CAD build for the part. Positions are in the model's coordinates, mm. Face numbers are marked on the shaded views. Round coordinates to 2 decimals unless told otherwise and drop trailing zeros. Loops run counter-clockwise (first coordinate to the right, second up) from the corner with the lowest first, then second, coordinate; pieces in that order, holes last.
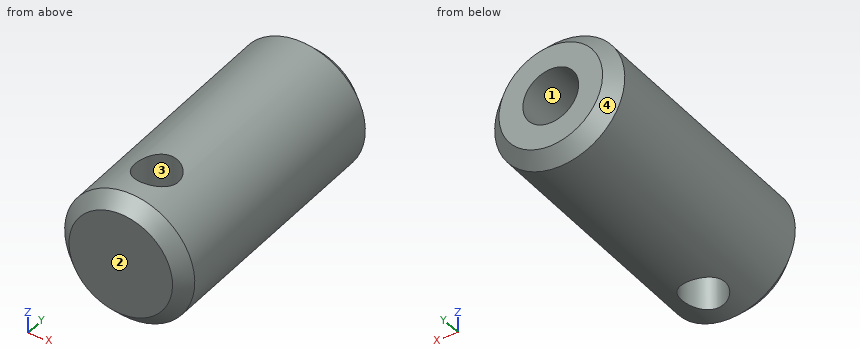
from build123d import *

# Parameters (mm, degrees)
SKETCH_1_R             = 4.9
EXTRUDE_1_DEPTH        = 21
HOLE_WIZARD_M4_1_D     = 3.3
HOLE_WIZARD_M5_1_D     = 4.2
HOLE_WIZARD_M5_1_DEPTH = 12
HOLE_WIZARD_M5_1_TIP   = 1.2618073
CHAMFER_1_SIZE         = 1


with BuildPart() as part:
    # 草图1 → 凸台-拉伸1 (new body)
    with BuildSketch(Plane(origin=(0, 0, 0), x_dir=(1, 0, 0), z_dir=(0, 1, 0))):
        with Locations(Location((0, 0, 0), (0, 0, 90))):
            Circle(SKETCH_1_R)
    extrude(amount=EXTRUDE_1_DEPTH)

    # M4 螺纹孔1 (through all)
    with Locations(Plane.XY.offset(4.9)):
        with Locations((0, 4)):
            Hole(HOLE_WIZARD_M4_1_D / 2)

    # M5 螺纹孔1
    with Locations(Plane(origin=(0, 21, 0), x_dir=(1, 0, 0), z_dir=(0, 1, 0))):
        with Locations((0, 0)):
            Hole(HOLE_WIZARD_M5_1_D / 2, depth=HOLE_WIZARD_M5_1_DEPTH)
            with Locations((0, 0, -(HOLE_WIZARD_M5_1_DEPTH + HOLE_WIZARD_M5_1_TIP / 2))):  # 118° drill point
                Cone(0, HOLE_WIZARD_M5_1_D / 2, HOLE_WIZARD_M5_1_TIP, mode=Mode.SUBTRACT)

    # 倒角1
    chamfer_1_edges = [part.edges().sort_by_distance(p)[0] for p in [
        (0, 0, 4.9),
        (0, 21, 4.9),
    ]]
    chamfer(chamfer_1_edges, length=CHAMFER_1_SIZE)


solid = part.part
Item 1: Cut at B-B (y = 4). List the corners of the cut face in (x, z), plus the area to 3 significant figures.
Verdict:
outline: (-1.65, -4.61) - (-1.65, 4.61) arc R4.9 ccw to start; (1.65, -4.61) arc R4.9 ccw to (1.65, 4.61) - close
area: 43.7 mm2
Item 2: Cut at C-C (y = 6.75). List the corners of the cut face in (x, z), plus the area to 3 significant figures.
Verdict:
outline: circle Ø9.8 at (0, 0)
area: 75.4 mm2
Item 3: Flat gauge pin, fed straight in: P1, Ø3, axis at x = 2.5, y = 9, coming from the -Z side. Where does the tip first touch, or does it go through?
Verdict:
P1: stops at z = -4.8
Item 4: Wall check: L1, parallel to X at y = 4, z = 0.25; L2, parallel to Z at x = -0.25, y = 19.25; L3, parallel to X at y = 4, z = -2. Give the ranges that are in metal, low to high.
Verdict:
L1: x = -4.89 to -1.65, 1.65 to 4.89
L2: z = -4.89 to -2.09, 2.09 to 4.89
L3: x = -4.47 to -1.65, 1.65 to 4.47
Item 5: Cut at A-A (y = 12). List the corners of the cut face in (x, z), plus the area to 3 significant figures.
Verdict:
outline: circle Ø9.8 at (0, 0); hole circle Ø4.2 at (0, 0)
area: 61.6 mm2
Item 6: Mould opens along Y. For the marked faces 1, 2, 3 and 4 say: released by +Y, released by -Y, zero draft, split by the parting line, or undercut.
Verdict:
face 1: zero draft
face 2: released by -Y
face 3: undercut
face 4: released by +Y
